Read the model definition and answer for the solid it produces. Units are mm, in the model's axes. A direction names the side the tool comes from. Coordinates: 2 decimals unless noted, no trailing zeros. Loops run counter-clockwise (first coordinate to the right, second up) from the corner with the lowest first, then second, coordinate; pieces in that order, holes last.
Autodesk Inventor part; units mm, degrees
ref_plane "Work Plane1" through (0, 15.5, 0) normal (0, 1, 0) x (-1, 0, 0)
ref_plane "Work Plane3" through (5.8328, -0.5, -3.3972) normal (-0.5032861, 0, -0.8641199) x (-0.8641199, 0, 0.5032861)
ref_plane "Work Plane2" through (4.9905, -0.5, 2.8561) normal (-0.4967067, 0, 0.8679184) x (0.8679184, 0, 0.4967067)
sketch "Sketch1" plane through (0, 0, 0) normal (0, 0, 1) x (1, 0, 0)
  line L0 (-6.25, -13.5) -> (-6.75, -13.5)
  line L1 (-6.75, -13.5) -> (-6.75, 15.5)
  line L2 (-6.25, 16) -> (-6.25, 16)
  line L3 (-5.75, 15.5) -> (-5.75, -13)
  arc A0 (-6.25, -13.5) -> (-5.75, -13) centre (-6.25, -13) ccw
  arc A1 (-6.25, 16) -> (-6.75, 15.5) centre (-6.25, 15.5) ccw
  arc A2 (-5.75, 15.5) -> (-6.25, 16) centre (-6.25, 15.5) ccw
  line L4 (0, -19.545) -> (0, 22.045)
  point P0 (-5.75, -13.5)
  point P1 (-6.75, 16)
  point P2 (0, 0)
  dimension "d2" = 29.5
  dimension "d3" = 1
  dimension "d4" = 5.75
  dimension "d5" = 13.5
  dimension "d6" = 0.5
revolve "Revolution1" add sketch "Sketch1" angle 360 about axis through (0, -10, 0) along (0, 1, 0)
ref_plane "Work Plane1" through (0, 15.5, 0) normal (0, 1, 0) x (-1, 0, 0)
sketch "Sketch3" plane through (0, 15.5, 0) normal (0, 1, 0) x (-1, 0, 0)
  circle A0 centre (0, 0) radius 6.75 construction
  circle A1 centre (0, 0) radius 5.75 construction
  arc A2 (-5.8328, -3.3972) -> (-5.8584, 3.3528) centre (0, 0) ccw
  arc A3 (-4.9687, -2.8939) -> (-4.9905, 2.8561) centre (0, 0) ccw
  line L0 (-0.0608, 0.0348) -> (-0.0605, -0.0352)
  line L1 (0, 0) -> (-0.0608, 0.0348)
  line L2 (-4.9905, 2.8561) -> (-5.8584, 3.3528)
  line L3 (0, 0) -> (-0.0605, -0.0352)
  line L4 (-4.9687, -2.8939) -> (-5.8328, -3.3972)
  point P0 (-0.0584, 6.7497)
  point P1 (-0.0071, -6.75)
  point P2 (-0.0546, 5.7497)
  point P3 (-0.0085, -5.75)
  dimension "d22" = 60
ref_plane "Work Plane3" through (5.8328, -0.5, -3.3972) normal (-0.5032861, 0, -0.8641199) x (-0.8641199, 0, 0.5032861)
sketch "Sketch4" plane through (5.8328, -0.5, -3.3972) normal (-0.5032861, 0, -0.8641199) x (-0.8641199, 0, 0.5032861)
  arc A0 (1, 16) -> (0, 16) centre (0.5, 16) ccw construction
  line L0 (0, 0) -> (0, 16) construction
  line L1 (1, 16) -> (1, 0) construction
  line L2 (0, 12.15) -> (1, 12.15)
  line L3 (1, 12.15) -> (1, 12)
  line L4 (1, 12) -> (0, 12)
  line L5 (0, 12) -> (0, 12.15)
  line L6 (6.75, -18.9) -> (6.75, 22.4)
  point P0 (6.75, 0.5)
  dimension "d14" = 1
  dimension "d15" = 0.15
  dimension "d16" = 4.5
revolve "Revolution2" cut sketch "Sketch4" angle 15 about axis through (0, -10, 0) along (0, -1, 0)
ref_plane "Work Plane2" through (4.9905, -0.5, 2.8561) normal (-0.4967067, 0, 0.8679184) x (0.8679184, 0, 0.4967067)
sketch "Sketch5" plane through (4.9905, -0.5, 2.8561) normal (-0.4967067, 0, 0.8679184) x (0.8679184, 0, 0.4967067)
  arc A0 (1, 16) -> (0, 16) centre (0.5, 16) ccw construction
  line L0 (0, 0) -> (0, 16) construction
  line L1 (1, 16) -> (1, 0) construction
  line L2 (0, 12.15) -> (1, 12.15)
  line L3 (1, 12.15) -> (1, 12)
  line L4 (1, 12) -> (0, 12)
  line L5 (0, 12) -> (0, 12.15)
  line L6 (6.75, -18.9) -> (6.75, 22.4)
  line L7 (-5.75, -27.16) -> (-5.75, 30.66)
  point P0 (-5.75, 0.5)
  point P1 (6.75, 0.5)
  dimension "d18" = 1
  dimension "d19" = 0.15
  dimension "d20" = 4.5
revolve "Revolution3" cut sketch "Sketch5" angle 15 about axis through (0, -10, 0) along (0, 1, 0)
extrude "Extrusion2" cut sketch "Sketch3" along normal blind 0.5 and the other way blind 16 contours L4 A3 L2 A2
properties part number "ConnectorSocket"
Q1. A cutting plane is placed at C-C (y = -9). Give the vertices of the cut face in (x, z), then the cut area to 3 significant figures.
Findings below:
outline: circle Ø13.5 at (0, 0); hole circle Ø11.5 at (0, 0)
area: 39.3 mm2
Q2. A cutting plane is placed at D-D (y = 6). Give the vertices of the cut face in (x, z).
Findings below:
outline: (4.97, -2.89) - (5.83, -3.4) arc R6.75 ccw to (5.86, 3.35) - (4.99, 2.86) arc R5.75 cw to start
Q3. Determine the mould class of faces 1 (the face through (5.39, 13.8, -3.14)), 2 (the face through (6, 11.65, -2)), 3 (the face through (-5, -13.5, -4)), 4 (the face through (-6, -0.5, 2)) for opening direction Y: +Y half, -Y half, draft (parallel to the pull), parting line (faces both ways), or undercut.
Findings below:
face 1: draft
face 2: undercut
face 3: -Y half
face 4: +Y half
Q4. Straight lines are drawn through the part: probe 1 along Z at (x, y) = (0, -2); probe 2 along Z at (x, y) = (4.25, -9.75); probe 3 along X at (y, z) = (-11.75, 3). For each, find the intervals that lie inside material, in ascending order.
Findings below:
probe 1: z = -6.75 to -5.75, 5.75 to 6.75
probe 2: z = -5.24 to -3.87, 3.87 to 5.24
probe 3: x = -6.05 to -4.91, 4.91 to 6.05
Q5. A cutting plane is placed at A-A (z = 0). Give the vertices of the cut face in (x, y), then the cut area to 3 significant figures.
Findings below:
outline: (-6.75, -13.5) - (-6.25, -13.5) arc R0.5 ccw to (-5.75, -13) - (-5.75, -0.5) - (-6.75, -0.5) - close; (5.75, -13) arc R0.5 ccw to (6.25, -13.5) - (6.75, -13.5) - (6.75, 15.5) arc R0.5 ccw to (5.75, 15.5) - close
area: 42.3 mm2
Q6. Which of the six approach directions +Z, -Z, +X, -X, +Y, -Y give full straight-line access (tool end or side, diameter ignored) to faces 5 (the face through (5.39, 5.42, -3.14)), 6 (the face through (5.744, -5.283, -0.253)), 7 (the face through (5.42, 5.42, 3.1))?
Findings below:
face 5: -Z, -X, +Y
face 6: +Y, -Y
face 7: +Z, -X, +Y
Q7. A flat-ended cylindrical pin translates along its axis: pin 1 Ø5 at (x, y) = (2.5, 8) entering from -Z. Find the tip coordinate at first contact, or state that the pin passes through.
Findings below:
pin 1: stops at z = -2.91
Q8. A cutting plane is placed at B-B (x = 0). Give the vertices of the cut face in (y, z), then the cut area to 3 significant figures.
Findings below:
outline: (-13.5, -6.75) - (-0.5, -6.75) - (-0.5, -5.75) - (-13, -5.75) arc R0.5 ccw to (-13.5, -6.25) - close; (-13.5, 6.25) arc R0.5 ccw to (-13, 5.75) - (-0.5, 5.75) - (-0.5, 6.75) - (-13.5, 6.75) - close
area: 25.9 mm2
